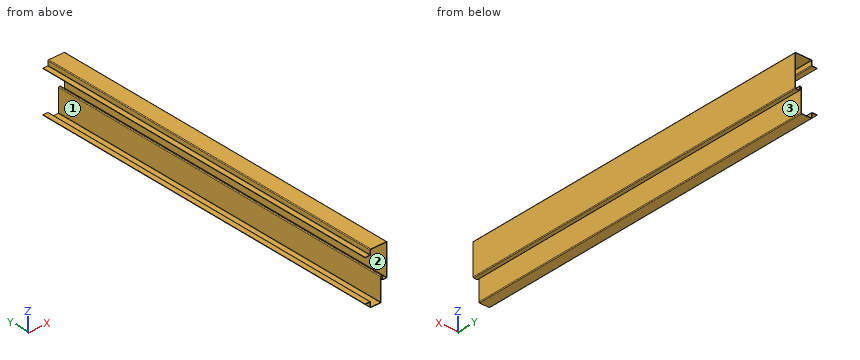
from build123d import *

# Parameters (mm, degrees)
BASE_FLANGE1_DEPTH = 490.75


# Sheet-metal steps are written as plain solids
with BuildPart() as part:
    # Sketch1 → Base-Flange1 (new, symmetric)
    with BuildSketch(Plane(origin=(0, 0, 0), x_dir=(1, 0, 0), z_dir=(0, 1, 0))):
        with BuildLine():
            Line((-4.25, 57.25), (8.7634, 57.25))
            ThreePointArc((8.7634, 57.25), (9.284254855, 57.465745145), (9.5, 57.9866))
            Line((9.5, 57.9866), (9.5, 69.0134))
            ThreePointArc((9.5, 69.0134), (10.081861668, 70.418138332), (11.4866, 71))
            Line((11.4866, 71), (37.5134, 71))
            ThreePointArc((37.5134, 71), (38.918138332, 70.418138332), (39.5, 69.0134))
            Line((39.5, 69.0134), (39.5, 17))
            Line((39.5, 17), (39.5, 8.562771629))
            ThreePointArc((39.5, 8.562771629), (39.724914644, 8.032905932), (40.262306969, 7.826620346))
            Line((40.262306969, 7.826620346), (42.153527557, 7.892663224))
            ThreePointArc((42.153527557, 7.892663224), (42.675221066, 8.135932903), (42.862626267, 8.680197126))
            Line((42.862626267, 8.680197126), (42.359529101, 15.874821789))
            ThreePointArc((42.359529101, 15.874821789), (42.88838258, 17.368257942), (44.341289843, 18))
            Line((44.341289843, 18), (53.5134, 18))
            ThreePointArc((53.5134, 18), (54.918138332, 17.418138332), (55.5, 16.0134))
            Line((55.5, 16.0134), (55.5, -22))
            Line((55.5, -22), (55.5, -67.0134))
            ThreePointArc((55.5, -67.0134), (54.918138332, -68.418138332), (53.5134, -69))
            Line((53.5134, -69), (39.5, -69))
            Line((39.5, -69), (11.4866, -69))
            ThreePointArc((11.4866, -69), (10.081861668, -68.418138332), (9.5, -67.0134))
            Line((9.5, -67.0134), (9.5, -55.9866))
            ThreePointArc((9.5, -55.9866), (9.284254855, -55.465745145), (8.7634, -55.25))
            Line((8.7634, -55.25), (-4.25, -55.25))
            Line((-4.25, -55.25), (-4.25, -54))
            Line((-4.25, -54), (8.7634, -54))
            ThreePointArc((8.7634, -54), (10.168138332, -54.581861668), (10.75, -55.9866))
            Line((10.75, -55.9866), (10.75, -67.0134))
            ThreePointArc((10.75, -67.0134), (10.965745145, -67.534254855), (11.4866, -67.75))
            Line((11.4866, -67.75), (39.5, -67.75))
            Line((39.5, -67.75), (53.5134, -67.75))
            ThreePointArc((53.5134, -67.75), (54.034254855, -67.534254855), (54.25, -67.0134))
            Line((54.25, -67.0134), (54.25, -22))
            Line((54.25, -22), (54.25, 16.0134))
            ThreePointArc((54.25, 16.0134), (54.034254855, 16.534254855), (53.5134, 16.75))
            Line((53.5134, 16.75), (44.341289843, 16.75))
            ThreePointArc((44.341289843, 16.75), (43.802574707, 16.515759992), (43.606484164, 15.962017381))
            Line((43.606484164, 15.962017381), (44.10958133, 8.767392718))
            ThreePointArc((44.10958133, 8.767392718), (43.604152098, 7.299519645), (42.197151928, 6.64342469))
            Line((42.197151928, 6.64342469), (40.30593134, 6.577381812))
            ThreePointArc((40.30593134, 6.577381812), (38.856591681, 7.133731182), (38.25, 8.562771629))
            Line((38.25, 8.562771629), (38.25, 17))
            Line((38.25, 17), (38.25, 69.0134))
            ThreePointArc((38.25, 69.0134), (38.034254855, 69.534254855), (37.5134, 69.75))
            Line((37.5134, 69.75), (11.4866, 69.75))
            ThreePointArc((11.4866, 69.75), (10.965745145, 69.534254855), (10.75, 69.0134))
            Line((10.75, 69.0134), (10.75, 57.9866))
            ThreePointArc((10.75, 57.9866), (10.168138332, 56.581861668), (8.7634, 56))
            Line((8.7634, 56), (-4.25, 56))
            Line((-4.25, 56), (-4.25, 57.25))
        make_face()
    extrude(amount=BASE_FLANGE1_DEPTH, both=True)


solid = part.part
The listing builds one solid part. Answer for the finished solid, in the listing's coordinates (mm). Face numbers are marked on the shaded views. Give positions to 0.01 mm unless a question says otherwise; leave off trailing zeros. Write each loop counter-clockwise with the first axis right and the second up, starting at its lowest first coordinate (ties: lowest second). Pieces come first, ordered by that corner, then holes.
Item 1: Determine the mould class of the marked faces 1, 2 and 3 for opening direction Z: released by +Z, released by -Z, zero draft, split by the parting line, or undercut.
Item 2: Flat-ended cylindrical pins translate along their axes: P1, Ø9, axis at y = 61.5, z = 64, coming from the -X side; P2, Ø12, axis at y = -117, z = -63.5, coming from the -X side; P3, Ø14.5, axis at x = 3.5, y = -79, coming from the +Z side; P4, Ø1.5, axis at x = 36, z = -6.5, coming from the -Y side. Find the tip coordinate at first contact, or state that the pin passes through.
Item 3: Find the intervals of material crossed by line 1 along X through (y, z) = (359, -62); line 2 along Z through (x, y) = (26, -353); line 3 along Z through (x, y) = (1.5, -342.5), in increasing order.
Item 4: Section A-A, the plane z = -40.5 is taken. Write down the section's boundary in (x, y), plus the area to 3 significant figures.
Completed:
1. face 1: undercut
1. face 2: undercut
1. face 3: zero draft
2. P1: stops at x = 9.5
2. P2: stops at x = 9.32
2. P3: stops at z = 68.86
2. P4: passes through
3. line 1: x = 9.5 to 10.75, 38.25 to 39.5
3. line 2: z = -71 to -69.75, 67.75 to 69
3. line 3: z = -57.25 to -56, 54 to 55.25
4. outline: (38.25, -490.75) - (39.5, -490.75) - (39.5, 490.75) - (38.25, 490.75) - close
4. area: 1,230 mm2
